Can you work these out from the model? Positions are in its coordinate system, mm. Face numbers are marked on the shaded views. A direction names the side the tool comes from. Round coordinates to 2 decimals unless told otherwise and drop trailing zeros. Order: outer loops, then holes, each group sorted by start corner. A loop starts at its lowest first (then second) coordinate and runs counter-clockwise, first axis right, second up. Notation, with made-up numbers: (31.5, 79) - (76.5, 79) arc R10 cw to (76.5, 98) - close; hole circle Ø8 at (64.5, 6.25). An arc over 180 degrees is marked (long way). Write item = value, one per line.
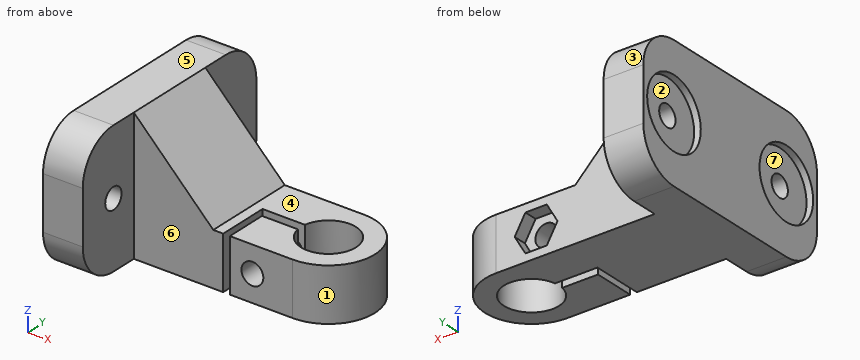
from build123d import *

# Parameters (mm, degrees)
RESSALTO_EXTRUS_O1_DEPTH   = 20
ESBO_O4_R                  = 1.6
CORTE_EXTRUS_O2_DEPTH      = 18
ESBO_O5_R                  = 5.25
CORTE_EXTRUS_O3_DEPTH      = 1
FILETE1_R                  = 6
CORTE_EXTRUS_O6_DEPTH      = 25
ESBO_O6_R                  = 1.65
CORTE_EXTRUS_O4_DEPTH      = 18.7
CORTE_EXTRUS_O4_DEPTH_BACK = 17.3
CORTE_EXTRUS_O5_DEPTH      = 2


with BuildPart() as part:
    # Esboço2 → Ressalto-extrusão1 (new body)
    with BuildSketch(Plane.XY):
        with BuildLine():
            Line((0, 7), (-24, 7))
            Line((-24, 7), (-24, 17))
            Line((-24, 17), (-30, 17))
            Line((-30, 17), (-30, -17))
            Line((-30, -17), (-24, -17))
            Line((-24, -17), (-24, -7))
            Line((-24, -7), (-10.5, -7))
            Line((-10.5, -7), (-10.5, 0.7))
            Line((-10.5, 0.7), (-4.090537862, 0.7))
            ThreePointArc((-4.090537862, 0.7), (4.15, 0), (-4.090537862, -0.7))
            Line((-4.090537862, -0.7), (-9.5, -0.7))
            Line((-9.5, -0.7), (-9.5, -7))
            Line((-9.5, -7), (0, -7))
            ThreePointArc((0, -7), (7, 0), (0, 7))
        make_face()
    extrude(amount=RESSALTO_EXTRUS_O1_DEPTH)

    # Esboço4 → Corte-extrusão2 (cut)
    with BuildSketch(Plane.ZY.offset(30)):
        with Locations((10, 11)):
            Circle(ESBO_O4_R)
        with Locations((10, -11)):
            Circle(ESBO_O4_R)
    extrude(amount=-CORTE_EXTRUS_O2_DEPTH, mode=Mode.SUBTRACT)

    # Esboço5 → Corte-extrusão3 (cut)
    with BuildSketch(Plane.ZY.offset(30)):
        with Locations((10, 11)):
            Circle(ESBO_O5_R)
        with Locations((10, -11)):
            Circle(ESBO_O5_R)
    extrude(amount=-CORTE_EXTRUS_O3_DEPTH, mode=Mode.SUBTRACT)

    # Filete1
    filete1_edges = [part.edges().sort_by_distance(p)[0] for p in [
        (-27, -17, 20),
        (-27, -17, 0),
        (-27, 17, 0),
        (-27, 17, 20),
    ]]
    fillet(filete1_edges, radius=FILETE1_R)

    # Esboço8 → Corte-extrusão6 (cut, through all)
    with BuildSketch(Plane(origin=(0, 7, 0), x_dir=(1, 0, 0), z_dir=(0, 1, 0))):
        Polygon((-24, -20), (-12, -8), (7, -8), (7, -20), align=None)
    extrude(amount=-CORTE_EXTRUS_O6_DEPTH, mode=Mode.SUBTRACT)

    # Esboço6 → Corte-extrusão4 (cut, two sides)
    with BuildSketch(Plane.XZ.offset(-0.7)) as corte_extrus_o4_sk:
        with Locations((-6.090537862, 4)):
            Circle(ESBO_O6_R)
    extrude(amount=CORTE_EXTRUS_O4_DEPTH, mode=Mode.SUBTRACT)
    extrude(corte_extrus_o4_sk.sketch, amount=-CORTE_EXTRUS_O4_DEPTH_BACK, mode=Mode.SUBTRACT)

    # Esboço7 → Corte-extrusão5 (cut)
    with BuildSketch(Plane(origin=(0, 7, 0), x_dir=(1, 0, 0), z_dir=(0, 1, 0))):
        Polygon((-2.857376354, -4), (-4.473957108, -1.2), (-7.707118616, -1.2), (-9.323699369, -4), (-7.707118616, -6.8), (-4.473957108, -6.8), align=None)
    extrude(amount=-CORTE_EXTRUS_O5_DEPTH, mode=Mode.SUBTRACT)


solid = part.part
(1) Thinking about a two-plate mould opening in Z: for the marked faces 1, 2 and 3, which applies, +Z half, -Z half, draft (parallel to the pull), parting line (faces both ways), or undercut?
Computed:
face_1 = draft
face_2 = undercut
face_3 = +Z half
(2) If we section it at C-C (x = -1.5): Write out the boundary of the cut face in (y, z).
Computed:
outline = (-7, 0) - (-3.87, 0) - (-3.87, 8) - (-7, 8) - close; (3.87, 0) - (7, 0) - (7, 8) - (3.87, 8) - close
(3) If we section it at B-B (y = -3.5): Write out the boundary of the cut face in (x, z).
Computed:
outline = (-30, 0) - (-10.5, 0) - (-10.5, 8) - (-12, 8) - (-24, 20) - (-30, 20) - close; (-9.5, 0) - (-2.23, 0) - (-2.23, 8) - (-9.5, 8) - close; (2.23, 0) - (6.06, 0) - (6.06, 8) - (2.23, 8) - close; hole circle Ø3.3 at (-6.09, 4)
(4) If we section it at A-A (y = 0): Write out the boundary of the cut face in (x, z).
Computed:
outline = (-30, 0) - (-10.5, 0) - (-10.5, 8) - (-12, 8) - (-24, 20) - (-30, 20) - close; (4.15, 0) - (7, 0) - (7, 8) - (4.15, 8) - close
(5) If I drill on line 1 (Y direction, x = -25.2, z = 10); line 2 (Y direction, x = -29.25, z = 10); line 3 (X direction, y = 0, z = 7.5), over which ranges is the centre line in solid material (lowest first)? Write a range as from..to.
Computed:
line_1 = -17..-12.6, -9.4..9.4, 12.6..17
line_2 = -17..-16.25, -5.75..5.75, 16.25..17
line_3 = -30..-10.5, 4.15..7
(6) Will these pins go through, and if not, where does the flat tip stop? P1, Ø2, axis at y = 12.5, z = 10, coming from the -X side; P2, Ø2, axis at x = -7, y = -1, coming from the +Z side; P3, Ø6, axis at x = -6.5, z = 3, coming from the +Y side.
Computed:
P1 = -29
P2 = 8
P3 = 7
(7) If we section it at D-D (z = 14.5): Write out the boundary of the cut face in (x, y), plus the area to 3 significant figures.
Computed:
outline = (-30, -16.98) - (-24, -16.98) - (-24, -7) - (-18.5, -7) - (-18.5, 7) - (-24, 7) - (-24, 16.98) - (-30, 16.98) - (-30, 13.7) - (-29, 13.7) - (-29, 8.3) - (-30, 8.3) - (-30, -8.3) - (-29, -8.3) - (-29, -13.7) - (-30, -13.7) - close
area = 270 mm^2
(8) On a 3-axis mill with a long thin cutter (end or side, diameter ignored), from which of +Z, -Z, +X, -X, +Y, -Y can I reach the whole of each face in a straight line? I mean the marked faces 4, 5, 6 and 7. Say none if no direction works.
Computed:
face_4 = +Z, +X, +Y, -Y
face_5 = +Z, +X, -X, +Y, -Y
face_6 = +Z, -Z, +X, -Y
face_7 = -X
